The model under review builds one solid part; all positions refer to its coordinate system, in mm. A direction names the side the tool comes from. Round coordinates to 2 decimals unless told otherwise and drop trailing zeros. Write each loop counter-clockwise with the first axis right and the second up, starting at its lowest first coordinate (ties: lowest second). Pieces come first, ordered by that corner, then holes. Notation, with made-up numbers: (27.25, 39) - (62.25, 39) arc R7 cw to (62.25, 52) - close; hole circle Ø1 at (12, -13.75). An arc over 180 degrees is marked (long way). Return JSON: item names as keys, results as strings.
from build123d import *

# Parameters (mm, degrees)
CUT_EXTRUDE_1_DEPTH      = 22.610182785
CUT_EXTRUDE_1_DEPTH_BACK = 22.610182785
SKETCH_3_W               = 3.8
SKETCH_3_H               = 4
SKETCH_4_R               = 1.75
CUT_EXTRUDE_2_DEPTH      = 4
CHAMFER_1_SIZE           = 1
CHAMFER_2_SIZE           = 0.2


with BuildPart() as part:
    # Эскиз2 → Повернуть1 (revolve)
    with BuildSketch(Plane(origin=(0, 0, 0), x_dir=(0, 0, -1), z_dir=(1, 0, 0)), mode=Mode.PRIVATE) as revolve_1_sk:
        Polygon((3.5, 15), (3.5, 0), (11, 0), (11, 4), (5.175, 4), (5.175, 15), align=None)
    revolve(revolve_1_sk.sketch.rotate(Axis((0, 40.815789474, 0), (0, -1, 0)), 180), axis=Axis((0, 40.815789474, 0), (0, -1, 0)))

    # Эскиз3 → Вырез-Вытянуть1 (cut, two sides: drawn at the far end of the back side and taken through both)
    with BuildSketch(Plane.XY.offset(-CUT_EXTRUDE_1_DEPTH_BACK)):
        with Locations((0, 13)):
            Rectangle(SKETCH_3_W, SKETCH_3_H)
    extrude(amount=CUT_EXTRUDE_1_DEPTH + CUT_EXTRUDE_1_DEPTH_BACK, mode=Mode.SUBTRACT)

    # Эскиз4 → Вырез-Вытянуть2 (cut)
    with BuildSketch(Plane.XZ):
        with Locations(Location((0, 8, 0), (0, 0, 270))):
            Circle(SKETCH_4_R)
        with Locations(Location((8, 0, 0), (0, 0, 270))):
            Circle(SKETCH_4_R)
        with Locations(Location((0, -8, 0), (0, 0, 270))):
            Circle(SKETCH_4_R)
        with Locations(Location((-8, 0, 0), (0, 0, 270))):
            Circle(SKETCH_4_R)
    extrude(amount=-CUT_EXTRUDE_2_DEPTH, mode=Mode.SUBTRACT)

    # Фаска1
    chamfer_1_edges = [part.edges().sort_by_distance(p)[0] for p in [
        (-3.5, 15, 0),
        (0, 0, -3.5),
        (3.5, 15, 0),
    ]]
    chamfer(chamfer_1_edges, length=CHAMFER_1_SIZE)

    # Фаска2
    chamfer_2_edges = [part.edges().sort_by_distance(p)[0] for p in [
        (-5.175, 15, 0),
        (0, 4, 9.75),
        (0, 0, 9.75),
        (8, 4, 1.75),
        (8, 0, 1.75),
        (5.175, 15, 0),
        (0, 4, -6.25),
        (0, 0, -6.25),
        (0, 4, -5.175),
        (-8, 4, 1.75),
        (-8, 0, 1.75),
        (0, 4, -11),
        (0, 0, -11),
    ]]
    chamfer(chamfer_2_edges, length=CHAMFER_2_SIZE)


solid = part.part
(1) Clearance check with flat-ended pins moving along their axes: pin 1 Ø2 at (y, z) = (13, 4) entering from -X; pin 2 Ø2 at (y, z) = (7, 5.5) entering from -X; pin 3 Ø3 at (y, z) = (6.5, -3.5) entering from -X. State where each tip first meets the part, or that it passes through.
Filled in:
{"pin 1": "stops at x = -4.22", "pin 2": "stops at x = -2.56", "pin 3": "stops at x = -4.77"}
(2) Add section B-B (x = 0). Give the number of separate pieces and of enclosed holes in the cut face, plus the area to 4 significant figures.
Filled in:
{"separate pieces": "4", "enclosed holes": "0", "area": "54.25 mm2"}
(3) Wall thickness on line 1 (X direction, y = 2.25, z = 0); line 2 (X direction, y = 8, z = 0) (3 decimals); line 3 (Z direction, x = -0.25, y = 3): over which ranges is each line inside the solid? List them lowest first.
Filled in:
{"line 1": "x = -11 to -9.75, -6.25 to -3.5, 3.5 to 6.25, 9.75 to 11", "line 2": "x = -5.175 to -3.5, 3.5 to 5.175", "line 3": "z = -11 to -9.73, -6.27 to -3.49, 3.49 to 6.27, 9.73 to 11"}
(4) Add section C-C (y = 9.5). Write out the cut boundary in (x, z) (3 decimals), plus the area to 3 significant figures.
Filled in:
{"outline": "circle Ø10.35 at (0, 0); hole circle Ø7 at (0, 0)", "area": "45.6 mm2"}
(5) Mouldability with a two-part tool opening along Z and no side actions: class faces 1 (the flat face through (-1.9, 13, -4)), 2 (the cylindrical face through (10.74, 2.03, -2.38)), 3 (the cylindrical face through (-0.154, 7.409, -3.497)) as released by +Z, released by -Z, zero draft, split by the parting line, or undercut.
Filled in:
{"face 1": "zero draft", "face 2": "split by the parting line", "face 3": "undercut"}
(6) Add section A-A (y = 3). Write out the cut boundary in (x, z).
Filled in:
{"outline": "circle Ø22 at (0, 0); hole circle Ø3.5 at (-8, 0); hole circle Ø7 at (0, 0); hole circle Ø3.5 at (0, -8); hole circle Ø3.5 at (0, 8); hole circle Ø3.5 at (8, 0)"}
(7) For faces 4 (the cylindrical face through (-0.67, 1.975, 6.383)), 5 (the flat face through (-1.9, 13, 4)), list the 3-axis set-ups (+Z, -Z, +X, -X, +Y, -Y) from which the entire face can be reached by the end or side of a thin tool; tool diameter is ignored.
Filled in:
{"face 4": "+Y, -Y", "face 5": "+Z, -Z, +Y"}
